```python
from build123d import *

# Parameters (mm, degrees)
SKETCH_1_W          = 71
SKETCH_1_H          = 40
EXTRUDE_1_DEPTH     = 93
EXTRUDE_START       = 35.5
SKETCH_2_W          = 39.063966261
SKETCH_2_H          = 60.96055705
SKETCH_2_R          = 1.986807663
SKETCH_2_R_2        = 2.303185406
SKETCH_2_R_3        = 2.435553703
SKETCH_2_R_4        = 2.279586572
EXTRUDE_2_DEPTH     = 2
CUT_EXTRUDE_1_DEPTH = 67


with BuildPart() as part:
    # 草图1 → 凸台-拉伸1 (new body)
    with BuildSketch(Plane.XY):
        Rectangle(SKETCH_1_W, SKETCH_1_H)
    extrude(amount=EXTRUDE_1_DEPTH)

    # 草图2 → 凸台-拉伸2 (add)
    with BuildSketch(Plane(origin=(0, 0, 0), x_dir=(0, 0, -1), z_dir=(1, 0, 0)).offset(EXTRUDE_START)):
        with Locations((-73.266758463, 0)):
            Rectangle(SKETCH_2_W, SKETCH_2_H)
        with Locations(Location((-87.266758464, 24.5, 0), (0, 0, 180))):
            Circle(SKETCH_2_R, mode=Mode.SUBTRACT)
        with Locations(Location((-59.266758464, 24.5, 0), (0, 0, 180))):
            Circle(SKETCH_2_R_2, mode=Mode.SUBTRACT)
        with Locations(Location((-87.266758464, -24.5, 0), (0, 0, 180))):
            Circle(SKETCH_2_R_3, mode=Mode.SUBTRACT)
        with Locations(Location((-59.266758464, -24.5, 0), (0, 0, 180))):
            Circle(SKETCH_2_R_4, mode=Mode.SUBTRACT)
    extrude(amount=EXTRUDE_2_DEPTH)

    # 草图3 → 切除-拉伸1 (cut)
    with BuildSketch(Plane(origin=(0, 20, 0), x_dir=(1, 0, 0), z_dir=(0, 1, 0))):
        Polygon((4.786467803, -93), (4.786467803, -32.304892778), (-35.5, -32.304892778), (-48.137036208, -34.916249884), (-56.319288473, -69.473208918), (-51.935451812, -90.687734689), (-39.693648232, -97.327684713), align=None)
    extrude(amount=-CUT_EXTRUDE_1_DEPTH, mode=Mode.SUBTRACT)


solid = part.part
```
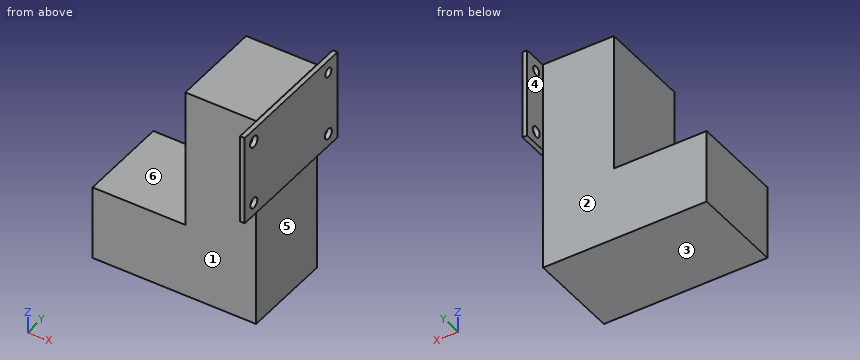
Geometry check sheet. Reference: the model listing, model coordinates, mm. Face numbers are marked on the shaded views. A direction names the side the tool comes from. Round coordinates to 2 decimals unless told otherwise and drop trailing zeros. Order: outer loops, then holes, each group sorted by start corner. A loop starts at its lowest first (then second) coordinate and runs counter-clockwise, first axis right, second up. Notation, with made-up numbers: (6, 42.25) -> (19, 42.25) arc R32 cw to (19, 76.25) -> close; hole circle Ø11 at (-16.5, 57). An arc over 180 degrees is marked (long way). Return JSON: item names as keys, results as strings. Group by question number.
Q1. Gauge pin test, flat ends, axial feed: pin 1 (8 mm diameter, centred on x = 13, y = 6, fed in from -Z); pin 2 (4 mm diameter, centred on y = 24.5, z = 59.27, fed in from +X); pin 3 (1 mm diameter, centred on x = 19, z = 26.5, fed in from +Y); pin 4 (20 mm diameter, centred on y = -5.5, z = 22.5, fed in from +X). Record the tip position at first contact, or that the pin passes through.
Q2. Section check B-B, the plane y = -24.5. Record the boundary of the cut face in (x, z), plus the area to 3 significant figures.
Q3. Tool access check on the marked faces 4, 5 and 6. Record the directions out of +Z, -Z, +X, -X, +Y, -Y that give a thin tool (end or side, any length) a straight path to the whole face; none if there is none.
Q4. Material ranges on probe 1 along Z at (x, y) = (36.6, -24.5); probe 2 along Z at (x, y) = (36.5, 24.5); probe 3 along X at (y, z) = (-19, 49), recorded low to high. Write a range as from..to.
Q5. Section check D-D, the plane x = 22. Record the boundary of the cut face in (y, z).
Q6. Section check A-A, the plane y = 24.5. Record the boundary of the cut face in (x, z).
Q7. Release check for a two-part mould opening along Y. For the marked faces 1, 2 and 3 record: released by +Y, released by -Y, zero draft, split by the parting line, or undercut.
Q8. Section check C-C, the plane z = 24.5. Record the boundary of the cut face in (x, y), plus the area to 3 significant figures.
Numbers:
{
 "1": {"pin 1": "z = 0", "pin 2": "through", "pin 3": "y = 20", "pin 4": "x = 35.5"},
 "2": {"outline": "(35.5, 53.73) -> (37.5, 53.73) -> (37.5, 56.99) -> (35.5, 56.99) -> close; (35.5, 61.55) -> (37.5, 61.55) -> (37.5, 84.83) -> (35.5, 84.83) -> close; (35.5, 89.7) -> (37.5, 89.7) -> (37.5, 92.8) -> (35.5, 92.8) -> close", "area": "59.3 mm^2"},
 "3": {"face 4": "+Z, -Z, -X, +Y", "face 5": "-Z, +X, +Y, -Y", "face 6": "+Z, -X, +Y, -Y"},
 "4": {"probe 1": "53.73..56.99, 61.55..84.83, 89.7..92.8", "probe 2": "53.73..56.96, 61.57..85.28, 89.25..92.8", "probe 3": "4.79..35.5"},
 "5": {"outline": "(-20, 0) -> (20, 0) -> (20, 93) -> (-20, 93) -> close"},
 "6": {"outline": "(35.5, 53.73) -> (37.5, 53.73) -> (37.5, 56.96) -> (35.5, 56.96) -> close; (35.5, 61.57) -> (37.5, 61.57) -> (37.5, 85.28) -> (35.5, 85.28) -> close; (35.5, 89.25) -> (37.5, 89.25) -> (37.5, 92.8) -> (35.5, 92.8) -> close"},
 "7": {"face 1": "released by -Y", "face 2": "released by +Y", "face 3": "zero draft"},
 "8": {"outline": "(-35.5, -20) -> (35.5, -20) -> (35.5, 20) -> (-35.5, 20) -> close", "area": "2,840 mm^2"}
}
